Work out the finished part from the listing and answer in its coordinate system (mm). A direction names the side the tool comes from. Round coordinates to 2 decimals unless told otherwise and drop trailing zeros. Order: outer loops, then holes, each group sorted by start corner. A loop starts at its lowest first (then second) coordinate and runs counter-clockwise, first axis right, second up. Notation, with made-up numbers: (68.25, 18) - (104.25, 18) arc R16 cw to (104.25, 45) - close; hole circle Ø11 at (56.25, 14). An arc over 180 degrees is marked (long way). Put each result on its own line as item: value.
```python
from build123d import *

# Parameters (mm, degrees)
SKETCH1_W           = 15
SKETCH1_H           = 2
BOSS_EXTRUDE1_DEPTH = 5
SKETCH1_3_W         = 1
SKETCH1_3_H         = 20
BOSS_EXTRUDE2_DEPTH = 5
LPATTERN1_COUNT     = 8
LPATTERN1_PITCH     = 2


with BuildPart() as part:
    # Sketch1 → Boss-Extrude1 (new body)
    with BuildSketch(Plane(origin=(0, 0, 0), x_dir=(1, 0, 0), z_dir=(0, 1, 0))):
        with Locations((1.806666667, -1.313333333)):
            Rectangle(SKETCH1_W, SKETCH1_H)
    extrude(amount=BOSS_EXTRUDE1_DEPTH)

    # Sketch1<3> → Boss-Extrude2 (add)
    with BuildSketch(Plane(origin=(0, 0, 0), x_dir=(1, 0, 0), z_dir=(0, 1, 0))):
        with Locations((-5.193333333, 9.686666667)):
            Rectangle(SKETCH1_3_W, SKETCH1_3_H)
    boss_extrude2 = extrude(amount=BOSS_EXTRUDE2_DEPTH)

    # LPattern1: Boss-Extrude2 ×8
    with Locations(*[(i * LPATTERN1_PITCH, 0, 0) for i in range(1, LPATTERN1_COUNT)]):
        add(boss_extrude2)


solid = part.part
```
1) A straight line is drawn through the part: L1, parallel to Z at x = -4, y = 2.1. Find the intervals that lie inside material, in ascending order. Write a range as from..to.
Findings below:
L1: z = 0.31..2.31
2) For faces 1 (the flat face through (6, 2, 0.313)), 2 (the flat face through (-5, 2, -19.687)), determine the directions among +Z, -Z, +X, -X, +Y, -Y from which every point of the face is accessible in a straight line to the end or side of a thin tool.
Findings below:
face 1: -Z, +Y, -Y
face 2: -Z, +X, -X, +Y, -Y
3) Given pin 1 Ø0.5 at (x, y) = (4, 2) entering from -Z; pin 2 Ø1 at (x, z) = (-3, -17) entering from -Y, each flat-ended and moving along its own axis, determine where each tip first touches the part or whether it passes through.
Findings below:
pin 1: stops at z = 0.31
pin 2: stops at y = 0
4) A cutting plane is placed at C-C on x = 6. Write down the section's boundary in (y, z), then the cut area to 3 significant figures.
Findings below:
outline: (0, 0.31) - (5, 0.31) - (5, 2.31) - (0, 2.31) - close
area: 10.0 mm2
5) For a pull along X with two mould halves and no side action, classify faces 3 (the flat face through (-1.693, 2, -10)), 4 (the flat face through (5, 2, -19.687)), 5 (the flat face through (9.307, 2, -9)) as pulls with the +X half, pulls with the -X half, needs draft (parallel to the pull), parting line crosses it, or undercut.
Findings below:
face 3: undercut
face 4: needs draft
face 5: pulls with the +X half
6) A cutting plane is placed at A-A on z = -1.5. Give the number of separate pieces and of enclosed holes in the cut face, then the cut area to 3 significant figures.
Findings below:
separate pieces: 8
enclosed holes: 0
area: 40.0 mm2
